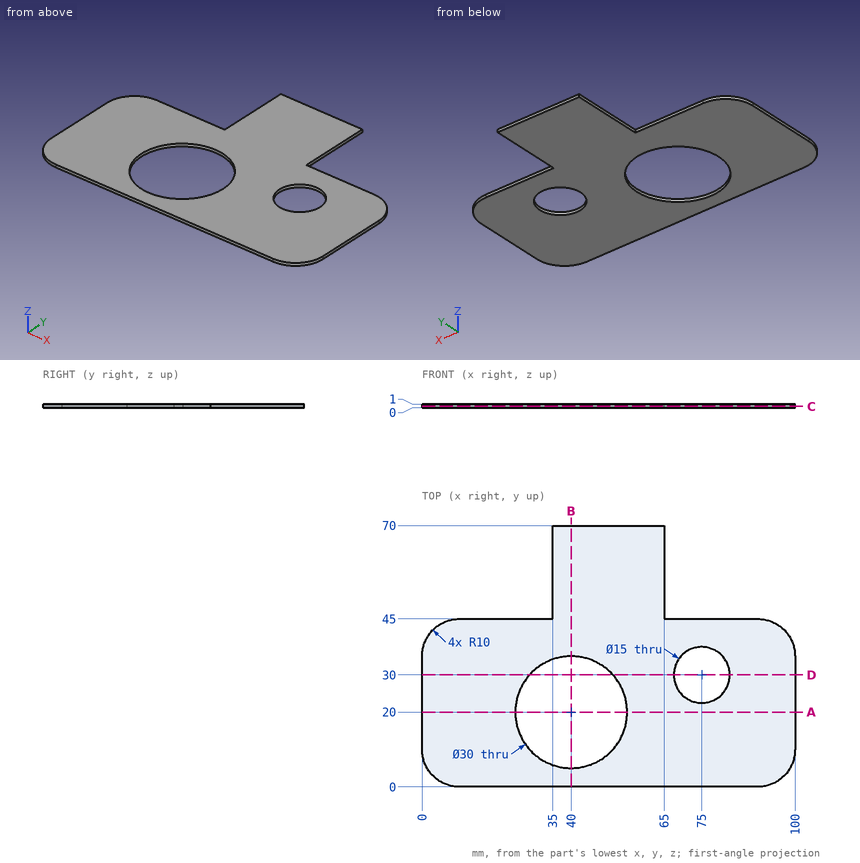
For this review, use the dimensioned drawing (mm, ordinates from the lowest corner) and the shaded views. Round coordinates to 2 decimals unless told otherwise and drop trailing zeros. Write each loop counter-clockwise with the first axis right and the second up, starting at its lowest first coordinate (ties: lowest second). Pieces come first, ordered by that corner, then holes. Notation, with made-up numbers: (26, 20.5) -> (82, 20.5) arc R22 ccw to (82, 44.5) -> close; hole circle Ø9 at (-2.5, -26.5). An arc over 180 degrees is marked (long way). Use one line per item in the form item = value.
Q1. Consider section D-D (y = 30). State the section outline as (x, z) points.
Resolved:
outline = (0, 0) -> (28.82, 0) -> (28.82, 1) -> (0, 1) -> close; (51.18, 0) -> (67.5, 0) -> (67.5, 1) -> (51.18, 1) -> close; (82.5, 0) -> (100, 0) -> (100, 1) -> (82.5, 1) -> close
Q2. Consider section A-A (y = 20). State the section outline as (x, z) points.
Resolved:
outline = (0, 0) -> (25, 0) -> (25, 1) -> (0, 1) -> close; (55, 0) -> (100, 0) -> (100, 1) -> (55, 1) -> close
Q3. To check wall thickness, follow probe 1 along Y at (x, z) = (40, 0.45); probe 2 along Y at (x, z) = (75, 0.65); probe 3 along Y at (x, z) = (88.5, 0.7). State the ranges of each line that lie inside material, in increasing order. Write a range as from..to.
Resolved:
probe_1 = 0..5, 35..70
probe_2 = 0..22.5, 37.5..45
probe_3 = 0..45
Q4. Consider section B-B (x = 40). State the section outline as (y, z) points.
Resolved:
outline = (0, 0) -> (5, 0) -> (5, 1) -> (0, 1) -> close; (35, 0) -> (70, 0) -> (70, 1) -> (35, 1) -> close
Q5. Clearance check with a flat-ended pin moving along its axis: pin 1 Ø0.5 at (y, z) = (62.5, 0.5) entering from -X. State where the tip first meets the part, or that it passes through.
Resolved:
pin_1 = 35
Q6. Consider section C-C (z = 0.35). State the section outline as (x, y) points.
Resolved:
outline = (0, 10) arc R10 ccw to (10, 0) -> (90, 0) arc R10 ccw to (100, 10) -> (100, 35) arc R10 ccw to (90, 45) -> (65, 45) -> (65, 70) -> (35, 70) -> (35, 45) -> (10, 45) arc R10 ccw to (0, 35) -> close; hole circle Ø30 at (40, 20); hole circle Ø15 at (75, 30)
